For this review, take the finished solid that the model builds, in its own axes (mm). A direction names the side the tool comes from. Give positions to 0.01 mm unless a question says otherwise; leave off trailing zeros. Write each loop counter-clockwise with the first axis right and the second up, starting at its lowest first coordinate (ties: lowest second). Pieces come first, ordered by that corner, then holes. Notation, with made-up numbers: (24.25, 73) -> (43.25, 73) arc R32 ccw to (43.25, 100) -> close; hole circle Ø6 at (54, 32). An arc over 180 degrees is marked (long way). Write item = value, one per line.
```python
from build123d import *

# Parameters (mm, degrees)
F0_R     = 3.15
F1_DEPTH = 1.2
F2_R     = 0.5


with BuildPart() as f1:
    # F0 (on Top) → F1 (new body)
    with BuildSketch(Plane.XY):
        Polygon((-4.5, 15), (0, 0), (18, 0), align=None)
        with BuildLine():
            Line((18, 0), (0, 0))
            Line((0, 0), (0, -12))
            Line((0, -12), (18, -12))
            ThreePointArc((18, -12), (24, -6), (18, 0))
        make_face()
        with Locations((6, -6)):
            Circle(F0_R, mode=Mode.SUBTRACT)
        with Locations((18, -6)):
            Circle(F0_R, mode=Mode.SUBTRACT)
        Polygon((18, -12), (0, -12), (-4.5, -27), align=None)
    extrude(amount=F1_DEPTH)

    # F2
    f2_edges = [f1.edges().sort_by_distance(p)[0] for p in [
        (-4.5, -27, 0.6),
        (-4.5, 15, 0.6),
    ]]
    fillet(f2_edges, radius=F2_R)


solid = f1.part
```
(1) For pin 1 (8 mm diameter, centred on x = 6, y = -6, fed in from +Z), flat-tipped, find the tip position at first contact; note if it passes through.
Answers below:
pin_1 = 1.2
(2) Take a section at A-A (y = -6). Write out the cut boundary in (x, z), plus the area to 3 significant figures.
Answers below:
outline = (0, 0) -> (2.85, 0) -> (2.85, 1.2) -> (0, 1.2) -> close; (9.15, 0) -> (14.85, 0) -> (14.85, 1.2) -> (9.15, 1.2) -> close; (21.15, 0) -> (24, 0) -> (24, 1.2) -> (21.15, 1.2) -> close
area = 13.7 mm^2
(3) Take a section at D-D (y = 11.5). Write out the cut boundary in (x, z).
Answers below:
outline = (-3.45, 0) -> (0.75, 0) -> (0.75, 1.2) -> (-3.45, 1.2) -> close
(4) Take a section at B-B (x = 6). Write out the cut boundary in (y, z), plus the area to 3 significant figures.
Answers below:
outline = (-20, 0) -> (-9.15, 0) -> (-9.15, 1.2) -> (-20, 1.2) -> close; (-2.85, 0) -> (8, 0) -> (8, 1.2) -> (-2.85, 1.2) -> close
area = 26.0 mm^2
(5) The part is to be moulded in two halves that separate along X. For faces 1 (the face through (-2.08, 6.93, 0.59)), 2 (the face through (24, -6, 1)), 3 (the face through (10, -6, 0)), 4 (the face through (14.853, -5.862, 0.592)), say which applies: released by +X, released by -X, zero draft, split by the parting line, or undercut.
Answers below:
face_1 = released by -X
face_2 = released by +X
face_3 = zero draft
face_4 = undercut
(6) Take a section at C-C (z = 0.65). Write out the cut boundary in (x, y).
Answers below:
outline = (-4.1, -25.67) arc R0.5 ccw to (-3.34, -26.23) -> (18, -12) arc R6 ccw to (18, 0) -> (-3.34, 14.23) arc R0.5 ccw to (-4.1, 13.67) -> (0, 0) -> (0, -12) -> close; hole circle Ø6.3 at (6, -6); hole circle Ø6.3 at (18, -6)
(7) To check wall thickness, follow probe 1 along X at (y, z) = (-8, 1.15); probe 2 along Y at (x, z) = (18, 0.45); probe 3 along Y at (x, z) = (8.75, 0.1). State the ranges of each line that lie inside material, in increasing order.
Answers below:
probe_1 = 0 to 3.57, 8.43 to 15.57, 20.43 to 23.66
probe_2 = -12 to -9.15, -2.85 to 0
probe_3 = -18.17 to -7.54, -4.46 to 6.17
(8) Tool access review of faces 5 (the face through (0, -6, 1)), 6 (the face through (9.005, -5.054, 0.592)): name each direction out of +Z, -Z, +X, -X, +Y, -Y from which nothing blocks a thin tool from reaching the whole face with its end or side.
Answers below:
face_5 = +Z, -Z, -X
face_6 = +Z, -Z
